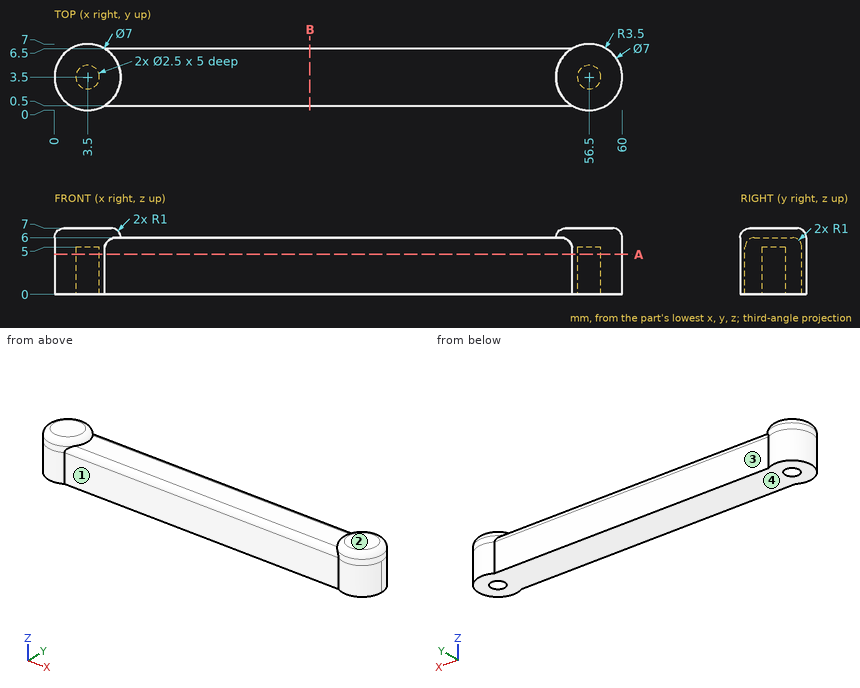
Here's the drawing with two shaded views (mm, measured from the low corner). I have some questions. A direction names the side the tool comes from. Round coordinates to 2 decimals unless told otherwise and drop trailing zeros. Write each loop counter-clockwise with the first axis right and the second up, starting at its lowest first coordinate (ties: lowest second). Pieces come first, ordered by that corner, then holes. Notation, with made-up numbers: M 89,34.25 L 134,34.25 A23 cw 134,52.25 Z; hole C -11,-23 d6. An arc over 180 degrees is marked long. Answer in a Markdown table with one row per item. Add a question column.
Q1. Imagine slicing it at B-B (x = 27). Please give me the cut outline in (y, z), then the cut area to 3 significant figures.
Q2. Will these pins go through, and if not, where does the flat tip stop? pin 1 Ø2 at (y, z) = (2, 3) entering from +X; pin 2 Ø1.5 at (x, z) = (30, 1.5) entering from +Y; pin 3 Ø3 at (x, y) = (43.5, 2) entering from +Z.
Q3. On a 3-axis mill with a long thin cutter (end or side, diameter ignored), from which of +Z, -Z, +X, -X, +Y, -Y can I reach the whole of each face in a straight line? I mean the marked faces 1 and 2. Say none if no direction works.
Q4. If I drill on line 1 (X direction, y = 3.25, z = 3); line 2 (X direction, y = 4.25, z = 4.5); line 3 (Y direction, x = 3.5, z = 3.6), over which ranges is the centre line in solid material (lowest first)? Write a range as from..to.
Q5. Imagine slicing it at A-A (z = 4.25). Please give me the cut outline in (x, y).
Q6. If we mould it in two halves opening along X, with no side actions, what happens to the marked faces 3 and 4? For each: +X half, -X half, draft (parallel to the pull), parting line (faces both ways), or undercut.
Values:
| question | item | result |
|---|---|---|
| 1 | outline | M 0.5,0 L 6.5,0 L 6.5,5 A1 ccw 5.5,6 L 1.5,6 A1 ccw 0.5,5 Z |
| 1 | area | 35.6 mm^2 |
| 2 | pin 1 | x = 59.96 |
| 2 | pin 2 | y = 6.5 |
| 2 | pin 3 | z = 6 |
| 3 | face 1 | +Z, -Z, -Y |
| 3 | face 2 | +Z, +X, -X, +Y, -Y |
| 4 | line 1 | 0.01..2.28, 4.72..55.28, 57.72..59.99 |
| 4 | line 2 | 0.08..2.5, 4.5..55.5, 57.5..59.92 |
| 4 | line 3 | 0..2.25, 4.75..7 |
| 5 | outline | M 5.3,0.5 L 54.7,0.5 A3.5 ccw long 54.7,6.5 L 5.3,6.5 A3.5 ccw long Z; hole C 3.5,3.5 d2.5; hole C 56.5,3.5 d2.5 |
| 6 | face 3 | undercut |
| 6 | face 4 | draft |
